Autodesk Inventor part; units mm, degrees
ref_plane "YZ Plane" through (0, 0, 0) normal (1, 0, 0) x (0, 1, 0)
ref_plane "XZ Plane" through (0, 0, 0) normal (0, 1, 0) x (-1, 0, 0)
ref_plane "XY Plane" through (0, 0, 0) normal (0, 0, 1) x (1, 0, 0)
sketch "Sketch1" plane through (0, 0, 0) normal (0, 0, 1) x (1, 0, 0)
  point P0 (0, 0)
sketch "Sketch2" plane through (0, 0, 0) normal (0, 1, 0) x (-1, 0, 0)
  line L0 (2.87, 0) -> (-2.87, 0)
  line L1 (0, -30) -> (0, 5)
  line L2 (2.05, 0) -> (-2.05, 0)
  line L3 (-2.05, 0) -> (-2.05, -25)
  line L4 (-2.05, -25) -> (2.05, -25)
  line L5 (2.05, -25) -> (2.05, 0)
  point P0 (0, 0)
  dimension "d0" = 4.1
  dimension "d1" = 25
sketch "Sketch2 outline for Extrusion1" plane through (0, 0, 0) normal (0, 1, 0) x (-1, 0, 0)
  line L0 (2.05, -25) -> (2.05, 0)
  line L1 (-2.05, -25) -> (2.05, -25)
  line L2 (-2.05, 0) -> (-2.05, -25)
  line L3 (2.05, 0) -> (-2.05, 0)
extrude "Extrusion1" add sketch "Sketch2 outline for Extrusion1" along normal blind 1.5 draft -5
sketch "Sketch3" plane through (0, 0, 0) normal (0, -1, 0) x (1, 0, 0)
  line L0 (-2.05, 0) -> (2.05, 0)
  line L1 (-2.05, -25) -> (-2.05, 0)
  line L2 (2.05, -25) -> (-2.05, -25)
  line L3 (2.05, 0) -> (2.05, -25)
  line L4 (-2.87, 0) -> (2.87, 0)
  line L5 (0, -30) -> (0, 5)
  line L6 (-2.05, 0) -> (2.05, 0)
  line L7 (2.05, 0) -> (0.25, 0)
  line L8 (0.25, 0) -> (0.25, -25)
  line L9 (0.25, -25) -> (2.05, -25)
  line L10 (2.05, -25) -> (2.05, 0)
  point P0 (0, 0)
  point P1 (0.25, 0)
  dimension "d4" = 1.8
extrude "Extrusion2" add sketch "Sketch3" along normal blind 0.035 contours L0 L3 L2 L8
mirror "Mirror1" about plane through (0, 0, 0) normal (1, 0, 0) of "Extrusion2"
sketch "Sketch4" plane through (0, -0.035, 0) normal (0, -1, 0) x (1, 0, 0)
  circle A0 centre (1.3, -2.5) radius 0.5
  line L0 (2.05, 0) -> (0.25, 0)
  line L1 (2.05, -25) -> (2.05, 0)
  point P0 (0, 0)
  dimension "d7" = 1
  dimension "d8" = 2.5
  dimension "d9" = 0.75
extrude "Extrusion3" cut sketch "Sketch4" against normal through all
pattern_linear "Rectangular Pattern1" count 9 spacing 2.5 along (0, 0, -1) count 2 spacing 2.5 along (-1, 0, 0) of "Extrusion3"
equation "\"BendRadius\" = Thickness"
equation "\"BendReliefWidth\" = Thickness"
equation "\"BendReliefDepth\" = 0.5 * Thickness"
equation "\"CornerReliefSize\" = 4 * Thickness"
equation "\"MinimumRemnant\" = 2 * Thickness"
equation "\"TransitionRadius\" = BendRadius"
equation "\"JacobiRadiusSize\" = BendRadius"
equation "\"GapSize\" = Thickness"
properties part number "VeroBoardLeadsSIngleHeater"
For this review, take the finished solid that the model builds, in its own axes (mm). Give positions to 0.01 mm unless a question says otherwise; leave off trailing zeros. Order: outer loops, then holes, each group sorted by start corner. A loop starts at its lowest first (then second) coordinate and runs counter-clockwise, first axis right, second up. Notation, with made-up numbers: (63, -17) - (73, -17) arc R25 cw to (73, -2) - close; hole circle Ø8 at (-10, 65.25). An arc over 180 degrees is marked (long way). Answer as a JSON object with one key per item and string values. Group by question number.
Item 1: Wall thickness on line 1 along Y through (x, z) = (0.2, -19.25); line 2 along Z through (x, y) = (-1.75, 1.25); line 3 along X through (y, z) = (1.3, -23.25): over which ranges is each line inside the solid? List them lowest first.
Item 2: Take a section at B-B on y = 0.95. Give the number of separate pieces and of enclosed holes in the cut face, and give its area (3 significant figures).
Item 3: Clearance check with a flat-ended pin moving along its axis: pin 1 Ø0.6 at (x, z) = (0, -14) entering from -Y (3 decimals). State where the tip first meets the part, or that it passes through.
Item 4: Take a section at C-C on z = -4. Give the boundary of the cut face in (x, y) (3 decimals).
Item 5: Draft analysis for pull direction Z (two halves, no side actions). For faces 1 (the flat face through (0.029, 0.739, -24.935)), 2 (the flat face through (-0.56, -0.035, -12.32)), 3 (the cylindrical face through (1.6, 0.7, -17.1)), state which applies: pulls with the +Z half, pulls with the -Z half, needs draft (parallel to the pull), parting line crosses it, or undercut.
Item 6: Take a section at A-A on z = -15. Give the boundary of the cut face in (x, y) (3 decimals), and give its area (3 significant figures).
Reported:
{
 "1": {"line 1": "0 to 1.5", "line 2": "-24.89 to -0.11", "line 3": "-1.94 to 1.94"},
 "2": {"separate pieces": "1", "enclosed holes": "18", "area": "83.6 mm^2"},
 "3": {"pin 1": "y = -0.035"},
 "4": {"outline": "(-2.05, -0.035) - (-0.25, -0.035) - (-0.25, 0) - (0.25, 0) - (0.25, -0.035) - (2.05, -0.035) - (2.05, 0) - (1.919, 1.5) - (-1.919, 1.5) - (-2.05, 0) - close"},
 "5": {"face 1": "pulls with the -Z half", "face 2": "needs draft", "face 3": "undercut"},
 "6": {"outline": "(-2.05, -0.035) - (-1.7, -0.035) - (-1.7, 1.5) - (-1.919, 1.5) - (-2.05, 0) - close; (-0.7, -0.035) - (-0.25, -0.035) - (-0.25, 0) - (0.25, 0) - (0.25, -0.035) - (0.8, -0.035) - (0.8, 1.5) - (-0.7, 1.5) - close; (1.8, -0.035) - (2.05, -0.035) - (2.05, 0) - (1.919, 1.5) - (1.8, 1.5) - close", "area": "3.01 mm^2"}
}
